Design review of the part shown in the three views and the two pictorial views. Dimensions are in mm from the part's minimum x, y and z. Coordinates: 2 decimals unless noted, no trailing zeros. Write each loop counter-clockwise with the first axis right and the second up, starting at its lowest first coordinate (ties: lowest second). Pieces come first, ordered by that corner, then holes. Notation, with made-up numbers: (31, -23.75) - (89, -23.75) arc R26 ccw to (89, -7.75) - close; hole circle Ø4 at (36.25, 80). An arc over 180 degrees is marked (long way). Answer as CSV lines item,"result". Start each with the question number.
Q1. We need section B-B (z = 2.4). Write out the cut boundary in (x, y).
Q2. We need section A-A (x = 53). Write out the cut boundary in (y, z).
Q3. Clearance check with flat-ended pins moving along their axes: pin 1 (2 mm diameter, centred on x = 53, z = 2, fed in from -Y); pin 2 (1.2 mm diameter, centred on y = 1.5, z = 2, fed in from +X). State where each tip first meets the part, or that it passes through.
Q4. We need section C-C (y = 23). Write out the cut boundary in (x, z).
Q5. We need section D-D (x = 41). Write out the cut boundary in (y, z).
Q6. For line 1 along X through (y, z) = (20, 1.95); line 2 along X through (y, z) = (3, 2.45); line 3 along Y through (x, z) = (55, 1.3), list the stretches that pass through material, from the lowest coordinate up. Write a range as [from, to].
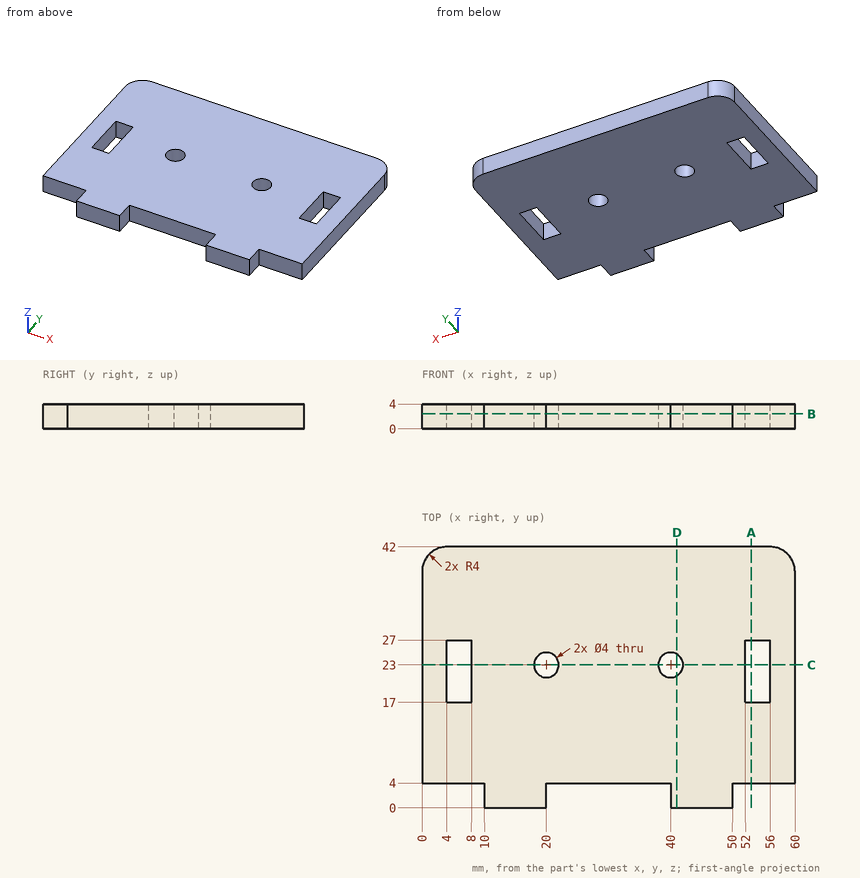
Results list:
1,outline,"(0, 4) - (10, 4) - (10, 0) - (20, 0) - (20, 4) - (40, 4) - (40, 0) - (50, 0) - (50, 4) - (60, 4) - (60, 38) arc R4 ccw to (56, 42) - (4, 42) arc R4 ccw to (0, 38) - close; hole (4, 17) - (8, 17) - (8, 27) - (4, 27) - close; hole circle Ø4 at (20, 23); hole circle Ø4 at (40, 23); hole (52, 17) - (56, 17) - (56, 27) - (52, 27) - close"
2,outline,"(4, 0) - (17, 0) - (17, 4) - (4, 4) - close; (27, 0) - (42, 0) - (42, 4) - (27, 4) - close"
3,pin 1,"stops at y = 4"
3,pin 2,"stops at x = 50"
4,outline,"(0, 0) - (4, 0) - (4, 4) - (0, 4) - close; (8, 0) - (18, 0) - (18, 4) - (8, 4) - close; (22, 0) - (38, 0) - (38, 4) - (22, 4) - close; (42, 0) - (52, 0) - (52, 4) - (42, 4) - close; (56, 0) - (60, 0) - (60, 4) - (56, 4) - close"
5,outline,"(0, 0) - (21.27, 0) - (21.27, 4) - (0, 4) - close; (24.73, 0) - (42, 0) - (42, 4) - (24.73, 4) - close"
6,line 1,"x = [0, 4], [8, 52], [56, 60]"
6,line 2,"x = [10, 20], [40, 50]"
6,line 3,"y = [4, 17], [27, 42]"
